For this review, take the finished solid that the model builds, in its own axes (mm). Face numbers are marked on the shaded views. A direction names the side the tool comes from. Give positions to 0.01 mm unless a question says otherwise; leave off trailing zeros. Order: outer loops, then holes, each group sorted by start corner. A loop starts at its lowest first (then second) coordinate and runs counter-clockwise, first axis right, second up. Notation, with made-up numbers: M 9,12 L 45,12 A27 ccw 45,43 Z; hole C 24.5,6 d6. An arc over 180 degrees is marked long. Answer as CSV lines item,"result". Start each with the question number.
1. For line 1 along Z through (x, y) = (-12.7, 83); line 2 along X through (y, z) = (81, -68); line 3 along Y through (x, z) = (27.5, -24.5), list the stretches that pass through material, from the lowest coordinate up.
2. Clearance check with flat-ended pins moving along their axes: P1, Ø6, axis at x = -1.5, y = 62.5, coming from the +Z side; P2, Ø4, axis at y = 50.5, z = -14, coming from the +X side; P3, Ø7, axis at y = 21, z = -15.5, coming from the +X side; P4, Ø7, axis at x = 64, z = -15.5, coming from the +Y side. State where each tip first meets the part, or that it passes through.
3. We need section B-B, the plane x = -12.7. Give the boundary of the cut face in (y, z).
4. We need section C-C, the plane z = -16.51. Give the boundary of the cut face in (x, y), and give its area (3 significant figures).
5. We need section D-D, the plane x = 52.5. Give the boundary of the cut face in (y, z).
6. We need section A-A, the plane y = 31.5. Give the boundary of the cut face in (x, z), and give its area (3 significant figures).
7. Mouldability with a two-part tool opening along X and no side actions: class the marked faces 1, 2 and 3 as pulls with the +X half, pulls with the -X half, needs draft (parallel to the pull), parting line crosses it, or undercut.
8. Machinability: for the marked faces 4, 5, 6, 7 and 8, which of the approach directions +Z, -Z, +X, -X, +Y, -Y give a long, thin tool a straight path to every point of the face, cutting with its end or side? Answer none if there is none.
Autodesk Inventor part; units mm, degrees
ref_plane "YZ Plane" through (0, 0, 0) normal (1, 0, 0) x (0, 1, 0)
ref_plane "XZ Plane" through (0, 0, 0) normal (0, 1, 0) x (-1, 0, 0)
ref_plane "XY Plane" through (0, 0, 0) normal (0, 0, 1) x (1, 0, 0)
sketch "Sketch1" plane through (0, 0, 0) normal (0, 1, 0) x (-1, 0, 0)
  line L0 (0, 0) -> (0, -85)
  line L1 (0, 0) -> (-60, 0)
  line L2 (-60, 0) -> (-60, -85)
  line L3 (-60, -85) -> (0, -85)
  line L4 (0, -42.5) -> (-76.2, -42.5)
  line L5 (-60, 0) -> (-66.35, 0)
  line L6 (-66.35, 0) -> (-66.35, -6.35)
  line L7 (-66.35, -6.35) -> (-60, -6.35)
  line L8 (-60, -6.35) -> (-60, 0)
  line L9 (0, 0) -> (6.35, 0)
  line L10 (6.35, 0) -> (6.35, -85)
  line L11 (6.35, -85) -> (0, -85)
  line L12 (-60, -85) -> (-66.35, -85)
  line L13 (-66.35, 0) -> (-76.2, -42.5)
  line L14 (-76.2, -42.5) -> (-66.35, -85)
  dimension "d0" = 85
  dimension "d1" = 60
  dimension "d2" = 76.2
  dimension "d3" = 6.35
  dimension "d4" = 6.35
  dimension "d5" = 6.35
  dimension "d6" = 6.35
extrude "Extrusion1" add sketch "Sketch1" along normal blind 12.7
sketch "Sketch2" plane through (0, 12.7, 0) normal (0, 1, 0) x (1, 0, 0)
  line L0 (-6.35, 0) -> (66.35, 0)
  line L1 (-6.35, 0) -> (-2.54, 0)
  line L2 (-2.54, 0) -> (-2.54, 3.81)
  line L3 (-2.54, 3.81) -> (-6.35, 3.81)
  line L4 (-6.35, 3.81) -> (-6.35, 0)
  line L5 (66.35, 85) -> (-6.35, 85)
  line L6 (-6.35, 85) -> (-2.54, 85)
  line L7 (-2.54, 85) -> (-2.54, 81.19)
  line L8 (-2.54, 81.19) -> (-6.35, 81.19)
  line L9 (-6.35, 81.19) -> (-6.35, 85)
  line L10 (66.35, 0) -> (62.54, 0)
  line L11 (62.54, 0) -> (62.54, 3.81)
  line L12 (62.54, 3.81) -> (66.35, 3.81)
  line L13 (66.35, 3.81) -> (66.35, 0)
  line L14 (66.35, 85) -> (62.54, 85)
  line L15 (62.54, 85) -> (62.54, 81.19)
  line L16 (62.54, 81.19) -> (66.35, 81.19)
  line L17 (66.35, 81.19) -> (66.35, 85)
  point P0 (0, 0)
  dimension "d9" = 3.81
  dimension "d10" = 3.81
  dimension "d11" = 3.81
  dimension "d12" = 3.81
  dimension "d13" = 3.81
  dimension "d14" = 3.81
  dimension "d15" = 3.81
  dimension "d16" = 3.81
extrude "Extrusion2" add sketch "Sketch2" along normal blind 12.7
sketch "Sketch3" plane through (-6.35, 0, -85) normal (-1, 0, 0) x (0, 0, 1)
  line L0 (3.81, 12.7) -> (81.19, 12.7)
  line L1 (42.5, 0) -> (0, 0)
  line L2 (81.19, 12.7) -> (3.81, 12.7)
  line L3 (3.81, 12.7) -> (3.81, 0)
  line L4 (3.81, 0) -> (81.19, 0)
  line L5 (81.19, 0) -> (81.19, 12.7)
  point P0 (85, 0)
extrude "Extrusion3" add sketch "Sketch3" along normal blind 12.7
sketch "Sketch4" plane through (0, 12.7, 0) normal (0, 1, 0) x (1, 0, 0)
  line L0 (-19.05, 3.81) -> (-19.05, 10.16)
  line L1 (-19.05, 81.19) -> (-19.05, 3.81)
  line L2 (-19.05, 10.16) -> (-6.35, 10.16)
  line L3 (-6.35, 10.16) -> (-6.35, 22.86)
  line L4 (-6.35, 22.86) -> (-19.05, 22.86)
  line L5 (-19.05, 22.86) -> (-19.05, 10.16)
  line L6 (-6.35, 81.19) -> (-19.05, 81.19)
  line L7 (-19.05, 81.19) -> (-19.05, 74.84)
  line L8 (-19.05, 74.84) -> (-6.35, 74.84)
  line L9 (-6.35, 74.84) -> (-6.35, 62.14)
  line L10 (-6.35, 62.14) -> (-19.05, 62.14)
  line L11 (-19.05, 62.14) -> (-19.05, 74.84)
  dimension "d39" = 6.35
  dimension "d40" = 12.7
  dimension "d41" = 12.7
  dimension "d42" = 6.35
  dimension "d43" = 12.7
  dimension "d44" = 12.7
extrude "Extrusion4" add sketch "Sketch4" along normal blind 76.2
sketch "Sketch5" plane through (0, 88.9, 0) normal (0, 1, 0) x (1, 0, 0)
  line L0 (-2.54, 3.81) -> (-6.35, 3.81)
  line L1 (-19.05, 74.84) -> (-19.05, 81.19)
  line L2 (-19.05, 74.84) -> (-19.05, 68.49)
  line L3 (-19.05, 81.19) -> (-19.05, 3.81)
  line L4 (-19.05, 68.49) -> (-12.7, 68.49)
  circle A0 centre (-12.7, 68.49) radius 3.81
  line L5 (-19.05, 22.86) -> (-19.05, 62.14)
  line L6 (-19.05, 22.86) -> (-19.05, 16.51)
  line L7 (-19.05, 16.51) -> (-12.7, 16.51)
  circle A1 centre (-12.7, 16.51) radius 3.81
  point P0 (0, 0)
  point P1 (-6.35, 68.49)
  dimension "d45" = 6.35
  dimension "d46" = 6.35
  dimension "d47" = 7.62
  dimension "d48" = 6.35
  dimension "d49" = 6.35
  dimension "d50" = 7.62
extrude "Extrusion5" cut sketch "Sketch5" against normal blind 12.7
sketch "Sketch6" plane through (0, 12.7, 0) normal (0, 1, 0) x (1, 0, 0)
  line L0 (62.54, 3.81) -> (66.35, 3.81)
  line L1 (66.35, 3.81) -> (66.35, 13.335)
  line L2 (66.35, 81.19) -> (62.54, 81.19)
  line L3 (66.35, 81.19) -> (66.35, 71.665)
  line L4 (66.35, 13.335) -> (60, 13.335)
  line L5 (60, 13.335) -> (60, 19.685)
  line L6 (60, 19.685) -> (66.35, 19.685)
  line L7 (66.35, 19.685) -> (66.35, 13.335)
  line L8 (66.35, 71.665) -> (60, 71.665)
  line L9 (60, 71.665) -> (60, 65.315)
  line L10 (60, 65.315) -> (66.35, 65.315)
  line L11 (66.35, 65.315) -> (66.35, 71.665)
  point P0 (0, 0)
  dimension "d31" = 9.525
  dimension "d32" = 9.525
  dimension "d33" = 6.35
  dimension "d34" = 6.35
  dimension "d35" = 6.35
  dimension "d36" = 6.35
extrude "Extrusion6" add sketch "Sketch6" along normal blind 12.7
properties part number "Maglev_Stand"
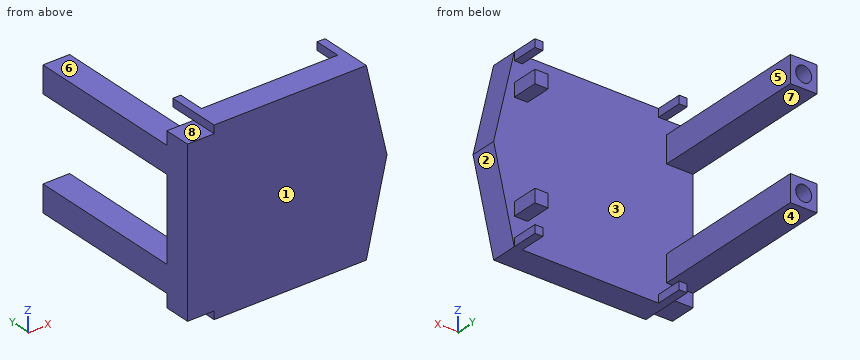
Result set:
1,line 1,"-74.84 to -72.3, -64.68 to -62.14, -22.86 to -20.32, -12.7 to -10.16"
1,line 2,"-19.05 to -16.48, -8.92 to -6.35"
1,line 3,"0 to 12.7"
2,P1,"through"
2,P2,"x = -6.35"
2,P3,"x = 66.35"
2,P4,"y = 25.4"
3,outline,"M 0,-81.19 L 12.7,-81.19 L 12.7,-74.84 L 88.9,-74.84 L 88.9,-72.3 L 76.2,-72.3 L 76.2,-64.68 L 88.9,-64.68 L 88.9,-62.14 L 12.7,-62.14 L 12.7,-22.86 L 88.9,-22.86 L 88.9,-20.32 L 76.2,-20.32 L 76.2,-12.7 L 88.9,-12.7 L 88.9,-10.16 L 12.7,-10.16 L 12.7,-3.81 L 0,-3.81 Z"
4,outline,"M -19.05,0 L 70.18,0 L 70.18,12.7 L 66.35,12.7 L 66.35,25.4 L 60,25.4 L 60,12.7 L -6.35,12.7 L -6.35,88.9 L -8.89,88.9 L -8.89,76.2 L -16.51,76.2 L -16.51,88.9 L -19.05,88.9 Z"
4,area,"2,080 mm2"
5,outline,"M 0,-85 L 12.7,-85 L 12.7,0 L 0,0 Z"
6,outline,"M -19.05,-74.84 L -6.35,-74.84 L -6.35,-62.14 L -19.05,-62.14 Z; M -19.05,-22.86 L -6.35,-22.86 L -6.35,-10.16 L -19.05,-10.16 Z"
6,area,"323 mm2"
7,face 1,"needs draft"
7,face 2,"pulls with the +X half"
7,face 3,"undercut"
8,face 4,"-Z, +X, -X, +Y"
8,face 5,"+Y"
8,face 6,"+Z, +X, -X, +Y"
8,face 7,"+X, -X, +Y"
8,face 8,"+Z, -X, +Y, -Y"
